from build123d import *

# Parameters (mm, degrees)
SKETCH_W        = 42
SKETCH_H        = 42
PAD_DEPTH       = 7
SKETCH001_R     = 11.5
POCKET_DEPTH    = 12
SKETCH002_R     = 1.75
POCKET001_DEPTH = 12
SKETCH003_R     = 1.9
POCKET002_DEPTH = 42
CHAMFER_SIZE    = 4


with BuildPart() as part:
    # Sketch → Pad (new body)
    with BuildSketch(Plane.XY):
        Rectangle(SKETCH_W, SKETCH_H)
    extrude(amount=PAD_DEPTH)

    # Sketch001 (on Face6 of Pad) → Pocket (cut)
    with BuildSketch(Plane.XY.offset(7)):
        Circle(SKETCH001_R)
    extrude(amount=-POCKET_DEPTH, mode=Mode.SUBTRACT)

    # Sketch002 (on Face5 of Pocket) → Pocket001 (cut)
    with BuildSketch(Plane.XY.offset(7)):
        with Locations((15.5, 15.5)):
            Circle(SKETCH002_R)
        with Locations((-15.5, 15.5)):
            Circle(SKETCH002_R)
        with Locations((-15.5, -15.5)):
            Circle(SKETCH002_R)
        with Locations((15.5, -15.5)):
            Circle(SKETCH002_R)
    extrude(amount=-POCKET001_DEPTH, mode=Mode.SUBTRACT)

    # Sketch003 (on Face1 of Pocket001) → Pocket002 (cut)
    with BuildSketch(Plane.XZ.offset(21)):
        with Locations((-10.25, 3.5)):
            Circle(SKETCH003_R)
        with Locations((10.25, 3.5)):
            Circle(SKETCH003_R)
    extrude(amount=-POCKET002_DEPTH, mode=Mode.SUBTRACT)

    # Chamfer
    chamfer_edges = [part.edges().sort_by_distance(p)[0] for p in [
        (-21, -21, 3.5),
        (21, -21, 3.5),
        (21, 21, 3.5),
        (-21, 21, 3.5),
    ]]
    chamfer(chamfer_edges, length=CHAMFER_SIZE)


solid = part.part
Design review of the part built by this model. Coordinates are the model's own, in mm. Round coordinates to 2 decimals unless told otherwise and drop trailing zeros. Loops run counter-clockwise (first coordinate to the right, second up) from the corner with the lowest first, then second, coordinate; pieces in that order, holes last. Notation, with made-up numbers: (25, -22.5) - (48, -22.5) arc R14 ccw to (48, 2.5) - close; hole circle Ø3 at (35, 26.5). An arc over 180 degrees is marked (long way). One line per item, written item: value. Start each with the question number.
1) Consider section B-B on z = 3.5. Give the boundary of the cut face in (x, y), then the cut area to 3 significant figures.
2) Draft analysis for pull direction Y (two halves, no side actions). For faces 1 (the cylindrical face through (15.272, 17.235, 3.549)), 2 (the cylindrical face through (-12.15, -0.29, 3.58)), 3 (the cylindrical face through (-14.6, 17, 3.5)), 4 (the flat face through (0, -21, 3)), state which applies: +Y half, -Y half, draft (parallel to the pull), parting line (faces both ways), or undercut.
3) Consider section C-C on y = 15.5. Give the boundary of the cut face in (x, z).
4) Consider section A-A on x = 0. Give the boundary of the cut face in (y, z), then the cut area to 3 significant figures.
5) Insertion check: pin 1 Ø4.5 at (x, y) = (15.5, -15.5) entering from -Z. The pin has a flat end and moves straight along its axis. Give the tip position at first contact, or say it passes through.
6) Consider section D-D on x = -15.5. Give the boundary of the cut face in (y, z).
7) To check wall thickness, follow L1, parallel to Y at x = 15.5, z = 3.75; L2, parallel to Y at x = -14, z = 2.25; L3, parallel to X at y = -6, z = 4. State the ranges of each line that lie inside material, in increasing order. Write a range as from..to.
Reported:
1. outline: (-21, -17) - (-17, -21) - (-12.15, -21) - (-12.15, 21) - (-17, 21) - (-21, 17) - close; (-8.35, -21) - (8.35, -21) - (8.35, -7.91) arc R11.5 cw to (-8.35, -7.91) - close; (-8.35, 7.91) arc R11.5 cw to (8.35, 7.91) - (8.35, 21) - (-8.35, 21) - close; (12.15, -21) - (17, -21) - (21, -17) - (21, 17) - (17, 21) - (12.15, 21) - close; hole circle Ø3.5 at (-15.5, -15.5); hole circle Ø3.5 at (-15.5, 15.5); hole circle Ø3.5 at (15.5, -15.5); hole circle Ø3.5 at (15.5, 15.5)
1. area: 1,030 mm^2
2. face 1: undercut
2. face 2: draft
2. face 3: undercut
2. face 4: -Y half
3. outline: (-21, 0) - (-17.25, 0) - (-17.25, 7) - (-21, 7) - close; (-13.75, 0) - (13.75, 0) - (13.75, 7) - (-13.75, 7) - close; (17.25, 0) - (21, 0) - (21, 7) - (17.25, 7) - close; hole circle Ø3.8 at (-10.25, 3.5); hole circle Ø3.8 at (10.25, 3.5)
4. outline: (-21, 0) - (-11.5, 0) - (-11.5, 7) - (-21, 7) - close; (11.5, 0) - (21, 0) - (21, 7) - (11.5, 7) - close
4. area: 133 mm^2
5. pin 1: stops at z = 0
6. outline: (-21, 0) - (-17.25, 0) - (-17.25, 7) - (-21, 7) - close; (-13.75, 0) - (13.75, 0) - (13.75, 7) - (-13.75, 7) - close; (17.25, 0) - (21, 0) - (21, 7) - (17.25, 7) - close
7. L1: y = -21..-17.25, -13.75..13.75, 17.25..21
7. L2: y = -21..-16.4, -14.6..14.6, 16.4..21
7. L3: x = -21..-12.08, 12.08..21
